Work out the finished part from the listing and answer in its coordinate system (mm). Face numbers are marked on the shaded views. A direction names the side the tool comes from. Coordinates: 2 decimals unless noted, no trailing zeros. Order: outer loops, then holes, each group sorted by start corner. A loop starts at its lowest first (then second) coordinate and runs counter-clockwise, first axis right, second up.
1. The part is cut by section C-C, the plane y = 35.5. Give the vertices of the cut face in (x, z).
2. The part is cut by section D-D, the plane x = -15.55. Give the vertices of the cut face in (y, z), then the cut area to 3 significant figures.
3. Flat-ended cylindrical pins translate along their axes: pin 1 Ø12.5 at (x, z) = (-10, 49) entering from +Y; pin 2 Ø5 at (x, z) = (15.55, 59) entering from +Y; pin 3 Ø0.9 at (x, z) = (-16, 59.5) entering from +Y; pin 4 Ø6 at (y, z) = (26, 52) entering from -X. Find the tip coordinate at first contact, or state that the pin passes through.
4. The part is cut by section A-A, the plane x = 0. Give the vertices of the cut face in (y, z), then the cut area to 3 significant figures.
5. The part is cut by section B-B, the plane z = 59. Give the vertices of the cut face in (x, y).
6. A tool of negligible diameter and unlimited length cuts with its end or side. For the marked faces 1 and 2, from which of +Z, -Z, +X, -X, +Y, -Y can it reach the whole face along a straight path? Write none if from no direction.
7. Find the intervals of material crossed by probe 1 along X at (y, z) = (22.95, 59); probe 2 along Z at (x, y) = (15.55, 24); probe 3 along Z at (x, y) = (-15, 23), in increasing order.
```python
from build123d import *

# Parameters (mm, degrees)
SKIZZE1_W                       = 42.3
SKIZZE1_H                       = 42.3
AUFSATZ_LINEAR_AUSTRAGEN1_DEPTH = 48
SKIZZE2_R                       = 11
AUFSATZ_LINEAR_AUSTRAGEN2_DEPTH = 2
SKIZZE3_R                       = 2.5
AUFSATZ_LINEAR_AUSTRAGEN3_DEPTH = 22
SKIZZE4_W                       = 5
SKIZZE4_H                       = 0.5
SCHNITT_LINEAR_AUSTRAGEN1_DEPTH = 15
SKIZZE6_R                       = 1.5
SCHNITT_LINEAR_AUSTRAGEN2_DEPTH = 4.5


with BuildPart() as part:
    # Skizze1 → Aufsatz-Linear austragen1 (new body)
    with BuildSketch(Plane.XZ.offset(-25)):
        with Locations((0, 43.45)):
            Rectangle(SKIZZE1_W, SKIZZE1_H)
    extrude(amount=AUFSATZ_LINEAR_AUSTRAGEN1_DEPTH)

    # Skizze2 → Aufsatz-Linear austragen2 (add)
    with BuildSketch(Plane(origin=(0, 25, 0), x_dir=(1, 0, 0), z_dir=(0, 1, 0))):
        with Locations(Location((0, -43.45, 0), (0, 0, 270))):
            Circle(SKIZZE2_R)
    extrude(amount=AUFSATZ_LINEAR_AUSTRAGEN2_DEPTH)

    # Skizze3 → Aufsatz-Linear austragen3 (add)
    with BuildSketch(Plane(origin=(0, 27, 0), x_dir=(1, 0, 0), z_dir=(0, 1, 0))):
        with Locations(Location((0, -43.45, 0), (0, 0, 270))):
            Circle(SKIZZE3_R)
    extrude(amount=AUFSATZ_LINEAR_AUSTRAGEN3_DEPTH)

    # Skizze4 → Schnitt-Linear austragen1 (cut)
    with BuildSketch(Plane(origin=(0, 49, 0), x_dir=(1, 0, 0), z_dir=(0, 1, 0))):
        with Locations((0, -41.2)):
            Rectangle(SKIZZE4_W, SKIZZE4_H)
    extrude(amount=-SCHNITT_LINEAR_AUSTRAGEN1_DEPTH, mode=Mode.SUBTRACT)

    # Skizze6 → Schnitt-Linear austragen2 (cut)
    with BuildSketch(Plane(origin=(0, 25, 0), x_dir=(1, 0, 0), z_dir=(0, 1, 0))):
        with Locations(Location((-15.55, -27.9, 0), (0, 0, 270))):
            Circle(SKIZZE6_R)
        with Locations(Location((-15.55, -59, 0), (0, 0, 270))):
            Circle(SKIZZE6_R)
    schnitt_linear_austragen2 = extrude(amount=-SCHNITT_LINEAR_AUSTRAGEN2_DEPTH, mode=Mode.SUBTRACT)

    # Spiegeln1: Schnitt-Linear austragen2 across plane
    add(schnitt_linear_austragen2.mirror(Plane.ZY), mode=Mode.SUBTRACT)


solid = part.part
```
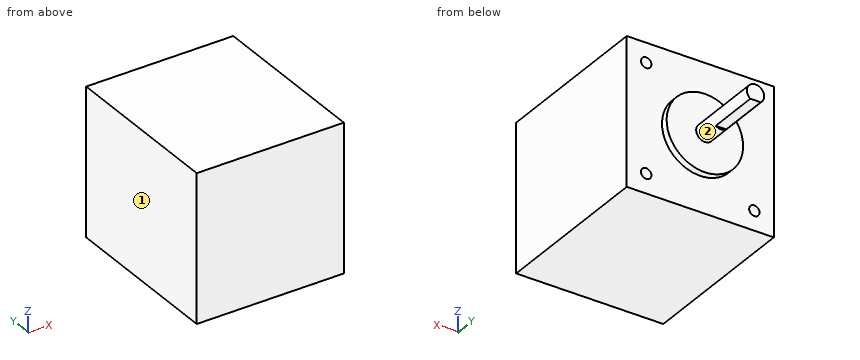
Geometry says:
1. outline: (-1.5, 41.45) - (1.5, 41.45) arc R2.5 ccw (long way) to start
2. outline: (-23, 22.3) - (25, 22.3) - (25, 26.4) - (20.5, 26.4) - (20.5, 29.4) - (25, 29.4) - (25, 57.5) - (20.5, 57.5) - (20.5, 60.5) - (25, 60.5) - (25, 64.6) - (-23, 64.6) - close
2. area: 2,000 mm2
3. pin 1: stops at y = 27
3. pin 2: stops at y = 25
3. pin 3: stops at y = 20.5
3. pin 4: stops at x = -21.15
4. outline: (-23, 22.3) - (25, 22.3) - (25, 32.45) - (27, 32.45) - (27, 40.95) - (34, 40.95) - (34, 41.45) - (49, 41.45) - (49, 45.95) - (27, 45.95) - (27, 54.45) - (25, 54.45) - (25, 64.6) - (-23, 64.6) - close
4. area: 2,180 mm2
5. outline: (-21.15, -23) - (21.15, -23) - (21.15, 25) - (17.05, 25) - (17.05, 20.5) - (14.05, 20.5) - (14.05, 25) - (-14.05, 25) - (-14.05, 20.5) - (-17.05, 20.5) - (-17.05, 25) - (-21.15, 25) - close
6. face 1: +Z, -Z, -X, +Y, -Y
6. face 2: +Y
7. probe 1: x = -21.15 to -17.05, -14.05 to 14.05, 17.05 to 21.15
7. probe 2: z = 22.3 to 26.4, 29.4 to 57.5, 60.5 to 64.6
7. probe 3: z = 22.3 to 26.5, 29.3 to 57.6, 60.4 to 64.6
